from build123d import *

# Parameters (mm, degrees)
SKETCH1_R                = 2.5
BOSS_EXTRUDE1_DEPTH      = 13
F_2_0_2_DIAMETER_HOLE1_D = 2
SKETCH8_R                = 1.5
CUT_EXTRUDE1_DEPTH       = 8


with BuildPart() as part:
    # Sketch1 → Boss-Extrude1 (new body)
    with BuildSketch(Plane.XY):
        with Locations(Location((0, 0, 0), (0, 0, 180))):
            Circle(SKETCH1_R)
    extrude(amount=BOSS_EXTRUDE1_DEPTH)

    # Sketch3 → Cut-Revolve1 (revolve, cut)
    with BuildSketch(Plane(origin=(0, 0, 0), x_dir=(1, 0, 0), z_dir=(0, 1, 0)), mode=Mode.PRIVATE) as cut_revolve1_sk:
        with BuildLine():
            Line((3.138230266, -4), (2.3, -4))
            ThreePointArc((2.3, -4), (2.017157288, -4.117157288), (1.9, -4.4))
            Line((1.9, -4.4), (1.9, -7.6))
            ThreePointArc((1.9, -7.6), (2.017157288, -7.882842712), (2.3, -8))
            Line((2.3, -8), (3.138230266, -8))
            Line((3.138230266, -8), (3.138230266, -4))
        make_face()
    revolve(cut_revolve1_sk.sketch.rotate(Axis((0, 0, 0), (0, 0, 1)), 180), axis=Axis((0, 0, 0), (0, 0, 1)), mode=Mode.SUBTRACT)

    # Ø2.0 (2) Diameter Hole1 (through all)
    with Locations(Plane.XY.offset(13)):
        with Locations((0, 0)):
            Hole(F_2_0_2_DIAMETER_HOLE1_D / 2)

    # Sketch8 → Cut-Extrude1 (cut)
    with BuildSketch(Plane.XY.offset(13)):
        Circle(SKETCH8_R)
    extrude(amount=-CUT_EXTRUDE1_DEPTH, mode=Mode.SUBTRACT)


solid = part.part
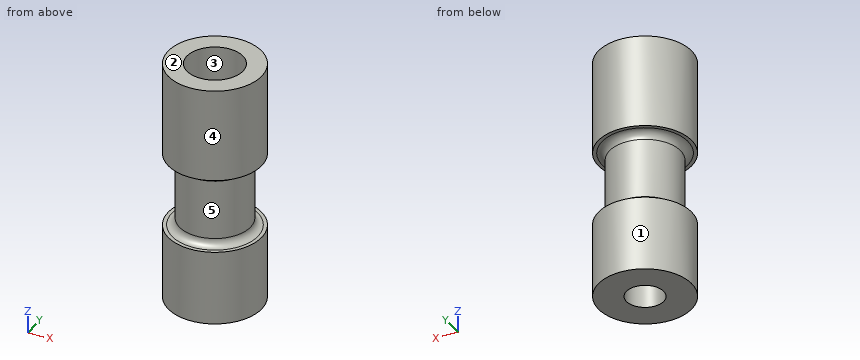
Geometry check sheet. Reference: the model listing, model coordinates, mm. Face numbers are marked on the shaded views. A direction names the side the tool comes from. Give positions to 0.01 mm unless a question says otherwise; leave off trailing zeros. Write each loop counter-clockwise with the first axis right and the second up, starting at its lowest first coordinate (ties: lowest second). Pieces come first, ordered by that corner, then holes.
1) Set-up check for the marked faces 4 and 5: record each of +Z, -Z, +X, -X, +Y, -Y from which the full face is reachable in a straight line by a thin tool's end or side.
Values follow:
face 4: +Z, -Z
face 5: none
2) Go/stop test with flat-tipped pins: pin 1 Ø0.9 at (x, y) = (0.5, 0) entering from +Z; pin 2 Ø1.5 at (y, z) = (-1.5, 7.5) entering from +X; pin 3 Ø1 at (x, y) = (0.5, 0.5) entering from +Z. Record where each tip stops, or that it passes through.
Values follow:
pin 1: passes through
pin 2: stops at x = 2.32
pin 3: stops at z = 5
3) Cross-section at C-C (z = 8.5). Record the boundary of the cut face in (x, y), plus the area to 3 significant figures.
Values follow:
outline: circle Ø5 at (0, 0); hole circle Ø3 at (0, 0)
area: 12.6 mm2
4) Cross-section at A-A (y = 0). Record the boundary of the cut face in (x, z), plus the area to 3 significant figures.
Values follow:
outline: (-2.5, 0) - (-1, 0) - (-1, 5) - (-1.5, 5) - (-1.5, 13) - (-2.5, 13) - (-2.5, 8) - (-2.3, 8) arc R0.4 cw to (-1.9, 7.6) - (-1.9, 4.4) arc R0.4 cw to (-2.3, 4) - (-2.5, 4) - close; (1, 0) - (2.5, 0) - (2.5, 4) - (2.3, 4) arc R0.4 cw to (1.9, 4.4) - (1.9, 7.6) arc R0.4 cw to (2.3, 8) - (2.5, 8) - (2.5, 13) - (1.5, 13) - (1.5, 5) - (1, 5) - close
area: 26.3 mm2
5) Release check for a two-part mould opening along X. For the marked faces 1, 2 and 3 record: released by +X, released by -X, zero draft, split by the parting line, or undercut.
Values follow:
face 1: split by the parting line
face 2: zero draft
face 3: undercut
6) Thickness scan on line 1 (Z direction, x = -0.15, y = 2.3); line 2 (Y direction, x = 0, z = 7); line 3 (Y direction, x = 0, z = 10). Record the ranges inside material, lowest first.
Values follow:
line 1: z = 0 to 4, 8 to 13
line 2: y = -1.9 to -1.5, 1.5 to 1.9
line 3: y = -2.5 to -1.5, 1.5 to 2.5
